```python
from build123d import *

# Parameters (mm, degrees)
SKETCH_1_R          = 8
EXTRUDE_1_DEPTH     = 3
HOLE_WIZARD_M31_D   = 3.4
HOLE_WIZARD_M51_D   = 5.5
HOLE_WIZARD_M52_D   = 5.5
FILLET_1_R          = 10
FILLET_2_R          = 5
CUT_EXTRUDE_1_DEPTH = 195.061830596
FILLET_3_R          = 4
SKETCH_9_R          = 9
CUT_EXTRUDE_2_DEPTH = 1
CUT_EXTRUDE_3_DEPTH = 195.061830596


with BuildPart() as part:
    # Эскиз1 → Бобышка-Вытянуть1 (new body)
    with BuildSketch(Plane.XY):
        with BuildLine():
            Line((-9.508526364, -3.096437692), (-1.398717752, -28))
            Line((-1.398717752, -28), (189.947361129, -28))
            ThreePointArc((189.947361129, -28), (191.995297124, 1.34383112), (189.536809823, 30.656120467))
            Line((189.536809823, 30.656120467), (125.388049295, 13.526041997))
            ThreePointArc((125.388049295, 13.526041997), (123.105499175, 12.698616461), (121.000225207, 11.489282104))
            Line((121.000225207, 11.489282104), (83.76563687, -14.436473614))
            Line((83.76563687, -14.436473614), (63.718090084, -22))
            Line((63.718090084, -22), (35.731449132, -22))
            Line((35.731449132, -22), (20.675178874, -13.02912429))
            Line((20.675178874, -13.02912429), (8.326583423, 5.537870395))
            ThreePointArc((8.326583423, 5.537870395), (-4.357415095, 9.00071851), (-9.508526364, -3.096437692))
        make_face()
        with Locations((129, 0)):
            Circle(SKETCH_1_R, mode=Mode.SUBTRACT)
    extrude(amount=EXTRUDE_1_DEPTH)

    # Отверстие с зазором M31 (through all)
    with Locations(Plane.XY.offset(3)):
        with Locations((9, -25), (40.5, -25), (72, -25)):
            Hole(HOLE_WIZARD_M31_D / 2)

    # Отверстие с зазором M51 (through all)
    with Locations(Plane.XY.offset(3)):
        with Locations((0, 0)):
            Hole(HOLE_WIZARD_M51_D / 2)

    # Отверстие с зазором M52 (through all)
    with Locations(Plane.XY.offset(3)):
        with Locations((183.228106674, 16.836297834), (183.914180714, 5.619086431), (183.914180714, -5.619086431), (183.228106674, -16.836297834)):
            Hole(HOLE_WIZARD_M52_D / 2)

    # Скругление1
    fillet_1_edges = [part.edges().sort_by_distance(p)[0] for p in [
        (35.731449132, -22, 1.5),
        (63.718090084, -22, 1.5),
        (83.76563687, -14.436473614, 1.5),
        (189.536809823, 30.656120467, 1.5),
        (189.947361129, -28, 1.5),
        (20.675178874, -13.02912429, 1.5),
    ]]
    fillet(fillet_1_edges, radius=FILLET_1_R)

    # Скругление2
    fillet_2_edges = [part.edges().sort_by_distance(p)[0] for p in [
        (-1.398717752, -28, 1.5),
    ]]
    fillet(fillet_2_edges, radius=FILLET_2_R)

    # Эскиз8 → Вырез-Вытянуть1 (cut, through all)
    with BuildSketch(Plane.XY.offset(3)):
        with BuildLine():
            Line((138.90792063, 9.891062066), (175.404223108, 19.636917172))
            ThreePointArc((175.404223108, 19.636917172), (176.470620047, 3.220288824), (176.003884761, -13.22431658))
            Line((176.003884761, -13.22431658), (138.90792063, 9.891062066))
        make_face()
        with BuildLine():
            Line((142.971746687, -0.888985098), (175.246255309, -21))
            Line((175.246255309, -21), (132.5, -21))
            Line((132.5, -21), (132.5, -13.555441712))
            ThreePointArc((132.5, -13.555441712), (139.790053932, -8.92046726), (142.971746687, -0.888985098))
        make_face()
        with BuildLine():
            Line((115.05010243, -1.183367143), (86.589440581, -21))
            Line((86.589440581, -21), (125.5, -21))
            Line((125.5, -21), (125.5, -13.555441712))
            ThreePointArc((125.5, -13.555441712), (118.304590303, -9.033726331), (115.05010243, -1.183367143))
        make_face()
    extrude(amount=-CUT_EXTRUDE_1_DEPTH, mode=Mode.SUBTRACT)

    # Скругление3
    fillet_3_edges = [part.edges().sort_by_distance(p)[0] for p in [
        (175.404223108, 19.636917172, 1.5),
        (176.003884761, -13.22431658, 1.5),
        (138.90792063, 9.891062066, 1.5),
        (115.05010243, -1.183367143, 1.5),
        (125.5, -13.555441712, 1.5),
        (125.5, -21, 1.5),
        (86.589440581, -21, 1.5),
        (175.246255309, -21, 1.5),
        (132.5, -21, 1.5),
        (132.5, -13.555441712, 1.5),
        (142.971746687, -0.888985098, 1.5),
    ]]
    fillet(fillet_3_edges, radius=FILLET_3_R)

    # Эскиз9 → Вырез-Вытянуть2 (cut)
    with BuildSketch(Plane(origin=(0, 0, 0), x_dir=(-1, 0, 0), z_dir=(0, 0, -1))):
        with Locations((-129, 0)):
            Circle(SKETCH_9_R)
    extrude(amount=-CUT_EXTRUDE_2_DEPTH, mode=Mode.SUBTRACT)

    # Эскиз10 → Вырез-Вытянуть3 (cut, through all)
    with BuildSketch(Plane.XY.offset(3)):
        with BuildLine():
            Line((6.5, -23.3), (11.5, -23.3))
            ThreePointArc((11.5, -23.3), (13.2, -25), (11.5, -26.7))
            Line((11.5, -26.7), (6.5, -26.7))
            ThreePointArc((6.5, -26.7), (4.8, -25), (6.5, -23.3))
        make_face()
        with BuildLine():
            Line((38, -23.3), (43, -23.3))
            ThreePointArc((43, -23.3), (44.7, -25), (43, -26.7))
            Line((43, -26.7), (38, -26.7))
            ThreePointArc((38, -26.7), (36.3, -25), (38, -23.3))
        make_face()
        with BuildLine():
            Line((69.5, -23.3), (74.5, -23.3))
            ThreePointArc((74.5, -23.3), (76.2, -25), (74.5, -26.7))
            Line((74.5, -26.7), (69.5, -26.7))
            ThreePointArc((69.5, -26.7), (67.8, -25), (69.5, -23.3))
        make_face()
    extrude(amount=-CUT_EXTRUDE_3_DEPTH, mode=Mode.SUBTRACT)


solid = part.part
```
Input: part model. Units: mm. Frame: model coordinates. A direction names the side the tool comes from. Give positions to 0.01 mm unless a question says otherwise; leave off trailing zeros. Loops run counter-clockwise (first coordinate to the right, second up) from the corner with the lowest first, then second, coordinate; pieces in that order, holes last.
1) Section query D-D on x = 51.5. Return the cut outline in (y, z), and give its area (3 significant figures).
A:
outline: (-28, 0) - (-22, 0) - (-22, 3) - (-28, 3) - close
area: 18.0 mm2
2) Section query B-B on y = 0. Return the cut outline in (x, z), and give its area (3 significant figures).
A:
outline: (-10, 0) - (-2.75, 0) - (-2.75, 3) - (-10, 3) - close; (2.75, 0) - (12.01, 0) - (12.01, 3) - (2.75, 3) - close; (104.5, 0) - (120, 0) - (120, 1) - (121, 1) - (121, 3) - (104.5, 3) - close; (137, 1) - (138, 1) - (138, 0) - (154.78, 0) - (154.78, 3) - (137, 3) - close; (176.5, 0) - (192, 0) - (192, 3) - (176.5, 3) - close
area: 197 mm2
3) Section query C-C on z = 1.55. Count the separate pieces of the cut face and the enclosed holes in it, and give its area (3 significant figures).
A:
separate pieces: 1
enclosed holes: 12
area: 4,070 mm2
4) Line query: L1, parallel to X at y = -10.5, z = 2.7; L2, parallel to X at y = 3.5, z = 0.95; L3, parallel to Y at x = 159, z = 1.5. Output: solid intervals per line, ascending.
A:
L1: x = -7.1 to 18.99, 89.42 to 101.67, 119.74 to 138.26, 158.4 to 191.71
L2: x = -9.37 to 9.68, 109.53 to 120.71, 137.29 to 149.16, 176.47 to 182.16, 185.67 to 191.97
L3: y = -28 to -21, -10.88 to -2.63, 15.26 to 22.5
5) Section query A-A on x = 129. Return the cut outline in (y, z).
A:
outline: (-28, 0) - (-9, 0) - (-9, 1) - (-8, 1) - (-8, 3) - (-28, 3) - close; (8, 1) - (9, 1) - (9, 0) - (14.49, 0) - (14.49, 3) - (8, 3) - close
6) Mould query, pull axis Y, two halves, no side actions, for faces 1 (the flat face through (28.071, -17.436, 1.479)), 2 (the flat face through (159.176, 15.303, 1.521)), 3 (the flat face through (105, -6, 0)). Classes: released by +Y, released by -Y, zero draft, split by the parting line, or undercut.
A:
face 1: released by +Y
face 2: undercut
face 3: zero draft
7) Reachability of faces 4 (the flat face through (103.15, -0.94, 1.48)), 5 (the flat face through (158.669, -2.423, 1.521)) from +Z, -Z, +X, -X, +Y, -Y: full face, straight path, thin tool, end or side. Return the list, or none.
A:
face 4: +Z, -Z, +Y
face 5: +Z, -Z
8) Contact query for flat-ended pins moving along their axis: pin 1 (0.9 mm diameter, centred on x = 144, z = 1, fed in from +Y); pin 2 (1.5 mm diameter, centred on x = 49, z = 2, fed in from +Y); pin 3 (0.9 mm diameter, centred on x = 72, z = 1, fed in from +Y). Output: stop coordinate, or through.
A:
pin 1: stops at y = 18.62
pin 2: stops at y = -22
pin 3: stops at y = -18.71
